Input: part model. Units: mm. Frame: model coordinates. A direction names the side the tool comes from. Coordinates: 2 decimals unless noted, no trailing zeros. Loops run counter-clockwise (first coordinate to the right, second up) from the corner with the lowest first, then second, coordinate; pieces in that order, holes last.
Item 1: Pull-direction query (X, two-part tool) for faces 3 (the cylindrical face through (154.047, 7.562, 1.57)), 4 (the conical face through (152.414, 2.829, 0.172)), 5 (the flat face through (304, 3, 0)), 6 (the flat face through (0, 0, 0)); classes: released by +X, released by -X, zero draft, split by the parting line, or undercut.
Item 2: Contact query for flat-ended pins moving along their axis: P1, Ø3, axis at x = 121, z = 3.5, coming from the +Y side; P2, Ø10, axis at x = 247, y = -5.5, coming from the -Z side; P3, Ø8, axis at x = 47.5, z = 9, coming from the +Y side. Output: stop coordinate, or through.
Item 3: Ray query, line 1 along Y through (x, z) = (299, 0); line 2 along Y through (x, z) = (7.25, 0); line 3 along Z through (x, y) = (3.5, 5.3). Return the intervals inside material, ascending.
Item 4: Reachability of faces 1 (the cylindrical face through (149.872, -10.846, 2.408)), 2 (the cylindrical face through (300.451, 0.775, 2.461)) from +Z, -Z, +X, -X, +Y, -Y: full face, straight path, thin tool, end or side. Return the list, or none.
Item 5: Section A-A on x = 46. Return loops of the section in (y, z), and give its area (3 significant figures).
```python
from build123d import *

# Parameters (mm, degrees)
SKETCH1_R                            = 11.11
BOSS_EXTRUDE1_DEPTH                  = 304
F_3_0_3_DIAMETER_HOLE2_D             = 3
F_3_0_3_DIAMETER_HOLE2_DEPTH         = 11
F_3_0_3_DIAMETER_HOLE2_TIP           = 0.901290929
F_13_64_0_20313_DIAMETER_HOLE2_D     = 5.159502
F_13_64_0_20313_DIAMETER_HOLE2_DEPTH = 7
F_13_64_0_20313_DIAMETER_HOLE2_TIP   = 1.550070783
F_13_64_0_20313_DIAMETER_HOLE4_D     = 5.159502
F_13_64_0_20313_DIAMETER_HOLE4_DEPTH = 7
F_13_64_0_20313_DIAMETER_HOLE4_TIP   = 1.550070783
F_13_64_0_20313_DIAMETER_HOLE5_D     = 5.159502
F_13_64_0_20313_DIAMETER_HOLE5_DEPTH = 7
F_13_64_0_20313_DIAMETER_HOLE5_TIP   = 1.550070783
F_13_64_0_20313_DIAMETER_HOLE6_D     = 5.159502
F_13_64_0_20313_DIAMETER_HOLE6_DEPTH = 7
F_13_64_0_20313_DIAMETER_HOLE6_TIP   = 1.550070783


with BuildPart() as part:
    # Sketch1 → Boss-Extrude1 (new body)
    with BuildSketch(Plane(origin=(0, 0, 0), x_dir=(0, 0, -1), z_dir=(1, 0, 0))):
        Circle(SKETCH1_R)
    extrude(amount=BOSS_EXTRUDE1_DEPTH)

    # Ø3.0 (3) Diameter Hole2
    with Locations(Plane.ZY):
        with Locations((0, 5.3)):
            Hole(F_3_0_3_DIAMETER_HOLE2_D / 2, depth=F_3_0_3_DIAMETER_HOLE2_DEPTH)
            with Locations((0, 0, -(F_3_0_3_DIAMETER_HOLE2_DEPTH + F_3_0_3_DIAMETER_HOLE2_TIP / 2))):  # 118° drill point
                Cone(0, F_3_0_3_DIAMETER_HOLE2_D / 2, F_3_0_3_DIAMETER_HOLE2_TIP, mode=Mode.SUBTRACT)

    # 13/64 (0.20313) Diameter Hole2
    with Locations(Plane(origin=(0, 11.11, 0), x_dir=(1, 0, 0), z_dir=(0, 1, 0))):
        with Locations((152, 0)):
            Hole(F_13_64_0_20313_DIAMETER_HOLE2_D / 2, depth=F_13_64_0_20313_DIAMETER_HOLE2_DEPTH)
            with Locations((0, 0, -(F_13_64_0_20313_DIAMETER_HOLE2_DEPTH + F_13_64_0_20313_DIAMETER_HOLE2_TIP / 2))):  # 118° drill point
                Cone(0, F_13_64_0_20313_DIAMETER_HOLE2_D / 2, F_13_64_0_20313_DIAMETER_HOLE2_TIP, mode=Mode.SUBTRACT)

    # 13/64 (0.20313) Diameter Hole4
    with Locations(Plane(origin=(0, -5.555, -9.621542236), x_dir=(-1, 0, 0), z_dir=(0, -0.50000000000001, -0.8660254037844328))):
        with Locations((-76, 0)):
            Hole(F_13_64_0_20313_DIAMETER_HOLE4_D / 2, depth=F_13_64_0_20313_DIAMETER_HOLE4_DEPTH)
            with Locations((0, 0, -(F_13_64_0_20313_DIAMETER_HOLE4_DEPTH + F_13_64_0_20313_DIAMETER_HOLE4_TIP / 2))):  # 118° drill point
                Cone(0, F_13_64_0_20313_DIAMETER_HOLE4_D / 2, F_13_64_0_20313_DIAMETER_HOLE4_TIP, mode=Mode.SUBTRACT)

    # 13/64 (0.20313) Diameter Hole5
    with Locations(Plane(origin=(0, -5.555, 9.621542236), x_dir=(-1, 0, 0), z_dir=(0, -0.499999999999998, 0.8660254037844398))):
        with Locations((-228, 0)):
            Hole(F_13_64_0_20313_DIAMETER_HOLE5_D / 2, depth=F_13_64_0_20313_DIAMETER_HOLE5_DEPTH)
            with Locations((0, 0, -(F_13_64_0_20313_DIAMETER_HOLE5_DEPTH + F_13_64_0_20313_DIAMETER_HOLE5_TIP / 2))):  # 118° drill point
                Cone(0, F_13_64_0_20313_DIAMETER_HOLE5_D / 2, F_13_64_0_20313_DIAMETER_HOLE5_TIP, mode=Mode.SUBTRACT)

    # 13/64 (0.20313) Diameter Hole6
    with Locations(Plane(origin=(304, 0, 0), x_dir=(0, 0, -1), z_dir=(1, 0, 0))):
        with Locations((0, 0)):
            Hole(F_13_64_0_20313_DIAMETER_HOLE6_D / 2, depth=F_13_64_0_20313_DIAMETER_HOLE6_DEPTH)
            with Locations((0, 0, -(F_13_64_0_20313_DIAMETER_HOLE6_DEPTH + F_13_64_0_20313_DIAMETER_HOLE6_TIP / 2))):  # 118° drill point
                Cone(0, F_13_64_0_20313_DIAMETER_HOLE6_D / 2, F_13_64_0_20313_DIAMETER_HOLE6_TIP, mode=Mode.SUBTRACT)


solid = part.part
```
Results found:
1. face 3: undercut
1. face 4: undercut
1. face 5: released by +X
1. face 6: released by -X
2. P1: stops at y = 10.93
2. P2: stops at z = -11.1
2. P3: stops at y = 9.92
3. line 1: y = -11.11 to -2.58, 2.58 to 11.11
3. line 2: y = -11.11 to 3.8, 6.8 to 11.11
3. line 3: z = -9.76 to -1.5, 1.5 to 9.76
4. face 1: +X, -X
4. face 2: +X
5. outline: circle Ø22.22 at (0, 0)
5. area: 388 mm2
